from build123d import *

# Parameters (mm, degrees)
F0_W     = 114.3
F0_H     = 685.8
F1_DEPTH = 19.05
F3_D     = 15.0114
F3_DEPTH = 14.224
F3_TIP   = 4.5098795482
F5_D     = 8.001
F5_DEPTH = 25.4
F5_TIP   = 2.4037429064
F7_D     = 8.001
F7_DEPTH = 25.4
F7_TIP   = 2.4037429064


with BuildPart() as f1:
    # F0 (on Right) → F1 (new body)
    with BuildSketch(Plane.YZ):
        Rectangle(F0_W, F0_H)
    extrude(amount=F1_DEPTH)

    # F3
    with Locations(Plane.YZ.offset(19.05)):
        with Locations((-33.274, 292.1), (33.274, 292.1), (-33.274, 0), (33.274, 0), (33.274, -292.1), (-33.274, -292.1)):
            Hole(F3_D / 2, depth=F3_DEPTH)
            with Locations((0, 0, -(F3_DEPTH + F3_TIP / 2))):  # 118° drill point
                Cone(0, F3_D / 2, F3_TIP, mode=Mode.SUBTRACT)

    # F5
    with Locations(Plane(origin=(0, 57.15, 0), x_dir=(-1, 0, 0), z_dir=(0, 1, 0))):
        with Locations((-9.525, -292.1), (-9.525, 292.1), (-9.525, 0)):
            Hole(F5_D / 2, depth=F5_DEPTH)
            with Locations((0, 0, -(F5_DEPTH + F5_TIP / 2))):  # 118° drill point
                Cone(0, F5_D / 2, F5_TIP, mode=Mode.SUBTRACT)

    # F7
    with Locations(Plane.XZ.offset(57.15)):
        with Locations((9.525, 292.1), (9.525, 0), (9.525, -292.1)):
            Hole(F7_D / 2, depth=F7_DEPTH)
            with Locations((0, 0, -(F7_DEPTH + F7_TIP / 2))):  # 118° drill point
                Cone(0, F7_D / 2, F7_TIP, mode=Mode.SUBTRACT)


solid = f1.part
Input: part model. Units: mm. Frame: model coordinates. A direction names the side the tool comes from. Give positions to 0.01 mm unless a question says otherwise; leave off trailing zeros. Answer as a JSON object with one key per item and string values. Group by question number.
Q1. Set-up query: faces 1 (the face through (11.838, 26.115, 294.355)), 2 (the face through (9, 57.15, -5)). Return all of +Z, -Z, +X, -X, +Y, -Y with unobstructed straight access to the full face (end or side cutting, diameter ignored); none if empty.
Q2. Mould query, pull axis Z, two halves, no side actions, for faces 3 (the face through (9, -1, 342.9)), 4 (the face through (9, -1, -342.9)), 5 (the face through (19.05, -1, 5)), 6 (the face through (1.1, 33.97, 293.2)). Classes: pulls with the +Z half, pulls with the -Z half, needs draft (parallel to the pull), parting line crosses it, or undercut.
Q3. Line query: probe 1 along Z at (x, y) = (10.5, 42); probe 2 along Z at (x, y) = (14, -36); probe 3 along X at (y, z) = (-52, -292). Output: solid intervals per line, ascending.
Q4. First-contact query: pin 1 Ø9 at (x, z) = (9.525, -292.1) entering from +Y; pin 2 Ø9 at (y, z) = (-33.274, -292.1) entering from +X. Flat tips, straight axial feed; report the tip coordinate or a pass-through.
Results:
{
 "1": {"face 1": "+X", "face 2": "+Z, -Z, +X, -X, +Y"},
 "2": {"face 3": "pulls with the +Z half", "face 4": "pulls with the -Z half", "face 5": "needs draft", "face 6": "undercut"},
 "3": {"probe 1": "-342.9 to -295.98, -288.22 to -3.88, 3.88 to 288.22, 295.98 to 342.9", "probe 2": "-342.9 to -299.09, -285.11 to -6.99, 6.99 to 285.11, 299.09 to 342.9", "probe 3": "0 to 5.53, 13.52 to 19.05"},
 "4": {"pin 1": "y = 57.15", "pin 2": "x = 3.02"}
}
